from build123d import *

# Parameters (mm, degrees)
F0_W         = 52.4002
F0_H         = 3.175
F1_DEPTH     = 6.35
F2_T1_DEPTH  = 63.119
F3_T1_DEPTH  = 6.35
F3_T3_DEPTH  = 2.413
F3_T6_ANGLE  = 233.2969892374
F3_T8_ANGLE  = 233.2969892374
F3_T10_ANGLE = 233.2969892374
F3_T12_ANGLE = 233.2969892374


# Not quite as in the source:
# - a fillet or chamfer that OpenCascade refuses, or shapes differently, is made with other operations: its cross-section is extruded or revolved along the edge and cut away or added


with BuildPart() as f1:
    # F0 (on Top) → F1 (new body)
    with BuildSketch(Plane.XY):
        with BuildLine():
            Line((25.4, 4.7625), (-25.4, 4.7625))
            ThreePointArc((-25.4, 4.7625), (-27.6450640303, 3.8325640303), (-28.575, 1.5875))
            Line((-28.575, 1.5875), (-28.575, -1.5875))
            ThreePointArc((-28.575, -1.5875), (-27.6450640303, -3.8325640303), (-25.4, -4.7625))
            Line((-25.4, -4.7625), (25.4, -4.7625))
            ThreePointArc((25.4, -4.7625), (27.6450640303, -3.8325640303), (28.575, -1.5875))
            Line((28.575, -1.5875), (28.575, 1.5875))
            ThreePointArc((28.575, 1.5875), (27.6450640303, 3.8325640303), (25.4, 4.7625))
        make_face()
        Rectangle(F0_W, F0_H, mode=Mode.SUBTRACT)
    extrude(amount=F1_DEPTH)

    # F2: fillet of radius 2.4638 on 2 edges, made by hand

    # F2_s2 → F2_t1 (cut)
    with BuildSketch(Plane.YZ.offset(-31.5595)):
        with BuildLine():
            ThreePointArc((-4.7625, 3.8862), (-4.0408696875, 5.6283696875), (-2.2987, 6.35))
            Line((-2.2987, 6.35), (-4.7625, 6.35))
            Line((-4.7625, 6.35), (-4.7625, 3.8862))
        make_face()
        with BuildLine():
            ThreePointArc((4.7625, 3.8862), (4.0408696875, 5.6283696875), (2.2987, 6.35))
            Line((2.2987, 6.35), (4.7625, 6.35))
            Line((4.7625, 6.35), (4.7625, 3.8862))
        make_face()
    extrude(amount=F2_T1_DEPTH, mode=Mode.SUBTRACT)

    # F3: fillet of radius 0.381 on 6 edges, made by hand

    # F3_s2 → F3_t1 (join)
    with BuildSketch(Plane.XY):
        with BuildLine():
            ThreePointArc((-26.2001, 1.2065), (-26.0885076836, 1.4759076836), (-25.8191, 1.5875))
            Line((-25.8191, 1.5875), (-26.2001, 1.5875))
            Line((-26.2001, 1.5875), (-26.2001, 1.2065))
        make_face()
        with BuildLine():
            ThreePointArc((26.2001, 1.2065), (26.0885076836, 1.4759076836), (25.8191, 1.5875))
            Line((25.8191, 1.5875), (26.2001, 1.5875))
            Line((26.2001, 1.5875), (26.2001, 1.2065))
        make_face()
        with BuildLine():
            ThreePointArc((26.2001, -1.2065), (26.0885076836, -1.4759076836), (25.8191, -1.5875))
            Line((25.8191, -1.5875), (26.2001, -1.5875))
            Line((26.2001, -1.5875), (26.2001, -1.2065))
        make_face()
        with BuildLine():
            ThreePointArc((-25.8191, -1.5875), (-26.0885076836, -1.4759076836), (-26.2001, -1.2065))
            Line((-26.2001, -1.2065), (-26.2001, -1.5875))
            Line((-26.2001, -1.5875), (-25.8191, -1.5875))
        make_face()
    extrude(amount=F3_T1_DEPTH)

    # F3_s4 → F3_t3 (cut)
    with BuildSketch(Plane.XZ.offset(-1.2065)):
        with BuildLine():
            ThreePointArc((-26.2001, 5.969), (-26.3116923164, 6.2384076836), (-26.5811, 6.35))
            Line((-26.5811, 6.35), (-26.2001, 6.35))
            Line((-26.2001, 6.35), (-26.2001, 5.969))
        make_face()
        with BuildLine():
            ThreePointArc((26.2001, 5.969), (26.3116923164, 6.2384076836), (26.5811, 6.35))
            Line((26.5811, 6.35), (26.2001, 6.35))
            Line((26.2001, 6.35), (26.2001, 5.969))
        make_face()
    extrude(amount=F3_T3_DEPTH, mode=Mode.SUBTRACT)

    # F3_s5 → F3_t6 (revolve, cut)
    with BuildSketch(Plane.XZ.offset(-1.2065)):
        with BuildLine():
            ThreePointArc((26.5811, 6.35), (26.3116923164, 6.2384076836), (26.2001, 5.969))
            Line((26.2001, 5.969), (26.2001, 6.35))
            Line((26.2001, 6.35), (26.5811, 6.35))
        make_face()
    revolve(axis=Axis((25.8191, 1.2065, 6.35), (0, 0, 1)), revolution_arc=F3_T6_ANGLE, mode=Mode.SUBTRACT)

    # F3_s7 → F3_t8 (revolve, cut)
    with BuildSketch(Plane.XZ.offset(1.2065)):
        with BuildLine():
            ThreePointArc((26.5811, 6.35), (26.3116923164, 6.2384076836), (26.2001, 5.969))
            Line((26.2001, 5.969), (26.2001, 6.35))
            Line((26.2001, 6.35), (26.5811, 6.35))
        make_face()
    revolve(axis=Axis((25.8191, -1.2065, 6.35), (0, 0, -1)), revolution_arc=F3_T8_ANGLE, mode=Mode.SUBTRACT)

    # F3_s9 → F3_t10 (revolve, cut)
    with BuildSketch(Plane(origin=(-16.0182318513, 11.9409314764, 0), x_dir=(0, 0, 1), z_dir=(-0.8017442393, 0.5976672776, 0))):
        with BuildLine():
            ThreePointArc((6.35, -15.6365356326), (6.2384076836, -15.9059433163), (5.969, -16.0175356326))
            Line((5.969, -16.0175356326), (6.35, -16.0175356326))
            Line((6.35, -16.0175356326), (6.35, -15.6365356326))
        make_face()
    revolve(axis=Axis((-25.8191, -1.2065, 6.35), (0, 0, -1)), revolution_arc=F3_T10_ANGLE, mode=Mode.SUBTRACT)

    # F3_s11 → F3_t12 (revolve, cut)
    with BuildSketch(Plane.XZ.offset(-1.2065)):
        with BuildLine():
            ThreePointArc((-26.5811, 6.35), (-26.3116923164, 6.2384076836), (-26.2001, 5.969))
            Line((-26.2001, 5.969), (-26.2001, 6.35))
            Line((-26.2001, 6.35), (-26.5811, 6.35))
        make_face()
    revolve(axis=Axis((-25.8191, 1.2065, 6.35), (0, 0, -1)), revolution_arc=F3_T12_ANGLE, mode=Mode.SUBTRACT)


solid = f1.part
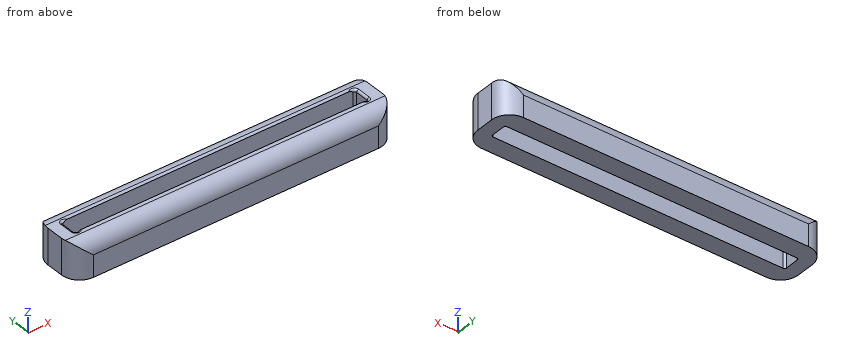
Read the model definition and answer for the solid it produces. Units are mm, in the model's axes. Give positions to 0.01 mm unless a question says otherwise; leave off trailing zeros. Write each loop counter-clockwise with the first axis right and the second up, starting at its lowest first coordinate (ties: lowest second). Pieces come first, ordered by that corner, then holes. Notation, with made-up numbers: (-36, 14.5) - (22, 14.5) arc R12 cw to (22, 30.5) - close; hole circle Ø1 at (25.5, 14). An arc over 180 degrees is marked (long way). Answer in a Markdown table with one row per item. Add a question column.
Item 1: Find the intervals of material crossed by L1, parallel to Y at x = -5, z = 1; L2, parallel to X at y = -1.25, z = 4.25 (3 decimals); L3, parallel to X at y = -2.25, z = 1.25, in increasing order.
Item 2: Section D-D, the plane y = 3.75 is taken. Write down the section's boundary in (x, z).
Item 3: Section B-B, the plane x = -5 is taken. Write down the section's boundary in (y, z), and give its area (3 significant figures).
Item 4: Section A-A, the plane y = -0.25 is taken. Write down the section's boundary in (x, z) (3 decimals), and give its area (3 significant figures).
Recorded:
| question | item | result |
|---|---|---|
| 1 | L1 | y = -4.76 to -1.59, 1.59 to 4.76 |
| 1 | L2 | x = -28.575 to -26.198, 26.198 to 28.575 |
| 1 | L3 | x = -28.51 to 28.51 |
| 2 | outline | (-27.72, 0) - (27.72, 0) - (27.72, 5.88) - (-27.72, 5.88) - close |
| 3 | outline | (-4.76, 0) - (-1.59, 0) - (-1.59, 6.35) - (-2.3, 6.35) arc R2.46 ccw to (-4.76, 3.89) - close; (1.59, 0) - (4.76, 0) - (4.76, 3.89) arc R2.46 ccw to (2.3, 6.35) - (1.59, 6.35) - close |
| 3 | area | 37.7 mm2 |
| 4 | outline | (-28.575, 0) - (-26.2, 0) - (-26.2, 5.969) arc R0.381 ccw to (-26.581, 6.35) - (-28.575, 6.35) - close; (26.2, 0) - (28.575, 0) - (28.575, 6.35) - (26.581, 6.35) arc R0.381 ccw to (26.2, 5.969) - close |
| 4 | area | 30.1 mm2 |
